Drawing for the job (mm, zero at the part's lowest x, y, z). Round coordinates to 2 decimals unless told otherwise and drop trailing zeros. Loops run counter-clockwise (first coordinate to the right, second up) from the corner with the lowest first, then second, coordinate; pieces in that order, holes last. Notation, with made-up numbers: M 66,51.5 L 78,51.5 A27 cw 78,77.5 Z; hole C -15.5,-35.75 d3. An arc over 180 degrees is marked long. Use a Markdown table: item, result. Add a question column.
Q1. Probe line 1 (X direction, y = 3, z = 7.25) (1 decimal); line 2 (Y direction, x = 6, z = 2.75) (1 decimal); line 3 (Y direction, x = 4.5, z = 6.25). List the from-to ranges inside material, lowest first. Write a range as from..to.
Q2. Pin check, flat tip, straight feed: pin 1 (1.5 mm diameter, centred on y = 6, z = 5, fed in from +X). Stop position of the tip, or through.
Q3. Cut at A-A (z = 5.5). Give the cut face in (x, y) (1 decimal), plus the area to 3 significant figures.
Q4. Cut at B-B (y = 2). Give the cut face in (x, z) (1 decimal).
Q5. Cut at C-C (x = 5.25). Give the cut face in (y, z).
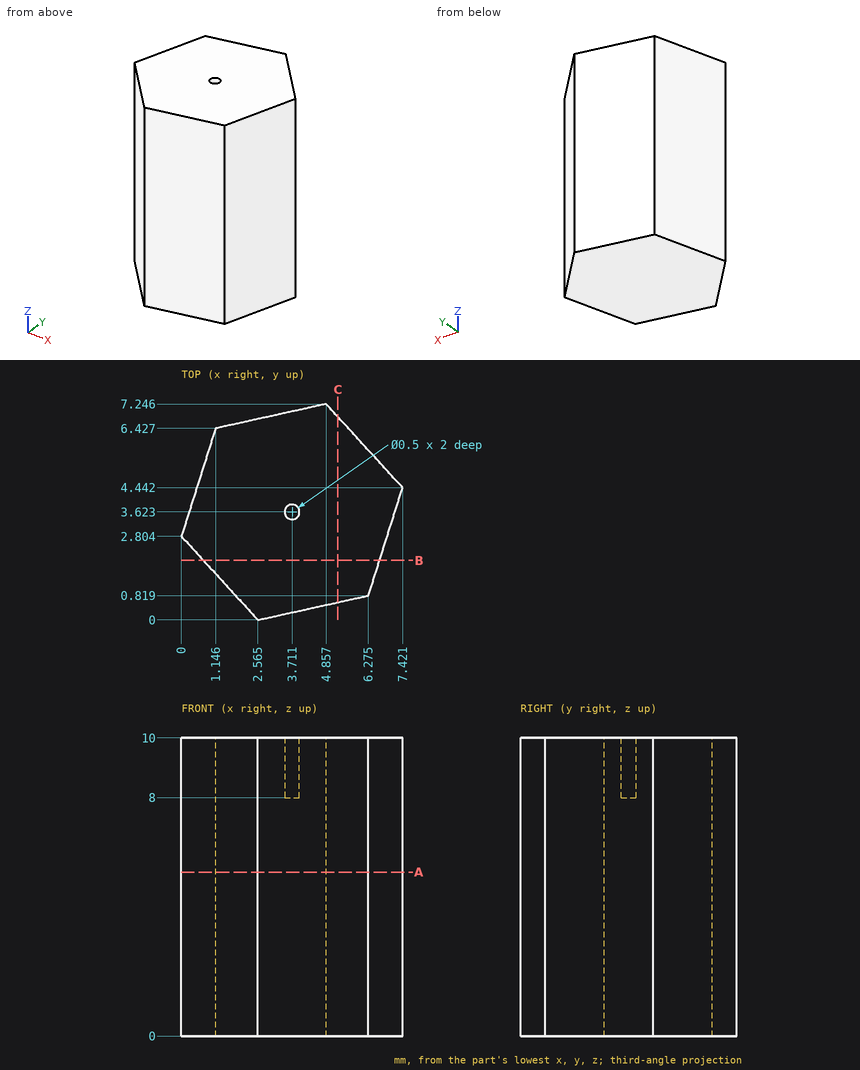
Checked values:
| question | item | result |
|---|---|---|
| 1 | line 1 | x = 0.1..7 |
| 1 | line 2 | y = 0.8..6 |
| 1 | line 3 | y = 0.43..7.17 |
| 2 | pin 1 | stops at x = 6.68 |
| 3 | outline | M 0,2.8 L 2.6,0 L 6.3,0.8 L 7.4,4.4 L 4.9,7.2 L 1.1,6.4 Z |
| 3 | area | 37.5 mm^2 |
| 4 | outline | M 0.7,0 L 6.6,0 L 6.6,10 L 0.7,10 Z |
| 5 | outline | M 0.59,0 L 6.82,0 L 6.82,10 L 0.59,10 Z |
